Autodesk Inventor part; units mm, degrees
ref_plane "YZ Plane" through (0, 0, 0) normal (1, 0, 0) x (0, 1, 0)
ref_plane "XZ Plane" through (0, 0, 0) normal (0, 1, 0) x (-1, 0, 0)
ref_plane "XY Plane" through (0, 0, 0) normal (0, 0, 1) x (1, 0, 0)
sketch "Sketch1" plane through (0, 0, 0) normal (1, 0, 0) x (0, 1, 0)
  circle A0 centre (0, 0) radius 3
  circle A1 centre (0, 77) radius 3
  circle A2 centre (36, 77) radius 3
  line L0 (-5, 78) -> (-5, -1)
  line L1 (-1, 82) -> (37, 82)
  line L2 (41, 78) -> (41, 76)
  line L3 (37, 72) -> (9, 72)
  line L4 (5, 68) -> (5, -1)
  line L5 (36, 77) -> (41, 77)
  line L6 (0, 0) -> (0, -5)
  line L7 (0, -5) -> (1, -5)
  line L8 (-1, -5) -> (0, -5)
  arc A3 (-1, 82) -> (-5, 78) centre (-1, 78) ccw
  arc A4 (-5, -1) -> (-1, -5) centre (-1, -1) ccw
  arc A5 (1, -5) -> (5, -1) centre (1, -1) ccw
  arc A6 (9, 72) -> (5, 68) centre (9, 68) ccw
  arc A7 (37, 72) -> (41, 76) centre (37, 76) ccw
  arc A8 (41, 78) -> (37, 82) centre (37, 78) ccw
  dimension "d0" = 6
  dimension "d1" = 77
  dimension "d3" = 10
  dimension "d4" = 5
  dimension "d5" = 4
  dimension "d6" = 10
  dimension "d9" = 46
extrude "Extrusion1" add sketch "Sketch1" along normal blind 19
sketch "Sketch3" plane through (0, 5, -1) normal (0, 1, 0) x (1, 0, 0)
  line L0 (19, 0) -> (19, -69)
  line L1 (19, -27) -> (0, -27)
  line L2 (0, -27) -> (0, -54)
  line L3 (0, -54) -> (19, -54)
  line L4 (19, -54) -> (19, -27)
  line L5 (0, 4) -> (19, 4)
  line L6 (0, -83) -> (19, -83)
  line L7 (0, 0) -> (0, -69)
  point P0 (0, -1)
  point P1 (19, -54)
  dimension "d15" = 31
  dimension "d16" = 29
extrude "Extrusion3" add sketch "Sketch3" along normal blind 8
fillet "Fillet1" radius 4 2 edges at (9.5, 5, 53) (9.5, 5, 26)
sketch "Sketch4" plane through (0, 5, -1) normal (0, 1, 0) x (1, 0, 0)
  line L0 (12.5, -15.2321) -> (9.5, -16.9641)
  line L1 (9.5, -16.9641) -> (6.5, -15.2321)
  line L2 (6.5, -15.2321) -> (6.5, -11.7679)
  line L3 (6.5, -11.7679) -> (9.5, -10.0359)
  line L4 (9.5, -10.0359) -> (12.5, -11.7679)
  line L5 (12.5, -11.7679) -> (12.5, -15.2321)
  line L6 (12.5, -65.2321) -> (9.5, -66.9641)
  line L7 (9.5, -66.9641) -> (6.5, -65.2321)
  line L8 (6.5, -65.2321) -> (6.5, -61.7679)
  line L9 (6.5, -61.7679) -> (9.5, -60.0359)
  line L10 (9.5, -60.0359) -> (12.5, -61.7679)
  line L11 (12.5, -61.7679) -> (12.5, -65.2321)
  line L12 (19, -58) -> (19, -69)
  line L13 (19, 0) -> (19, -23)
  line L14 (19, -23) -> (0, -23)
  line L15 (19, -27) -> (0, -27)
  line L16 (0, -54) -> (19, -54)
  circle A0 centre (9.5, -13.5) radius 1.5
  circle A1 centre (9.5, -63.5) radius 1.5
  point P0 (0, -1)
  point P1 (9.5, -23)
  dimension "d20" = 6
  dimension "d23" = 9.5
  dimension "d26" = 3
  dimension "d29" = 50
extrude "Extrusion4" cut sketch "Sketch4" against normal blind 3 contours L0 L1 L2 L3 L4 L5 | L6 L7 L8 L9 L10 L11 | A0 | A1
extrude "Extrusion5" cut sketch "Sketch4" against normal through all contours A0 | A1
sketch "Sketch5" plane through (0, 13, -1) normal (0, 1, 0) x (1, 0, 0)
  circle A0 centre (5.5, -31.8771) radius 1.25
  circle A1 centre (5.5, -48.8771) radius 1.25
  circle A2 centre (13.5, -31.8771) radius 1.25
  circle A3 centre (13.5, -48.8771) radius 1.25
  line L0 (19, -54) -> (19, -27)
  line L1 (0, -27) -> (0, -54)
  point P0 (0, -1)
  dimension "d30" = 2.5
  dimension "d31" = 17
  dimension "d32" = 5.5
  dimension "d33" = 5.5
extrude "Extrusion6" cut sketch "Sketch5" against normal through all
equation "\"d33\" = d32"
properties part number "wheel_mount"
Verification items for the finished model (mm, model axes). A direction names the side the tool comes from. Give positions to 0.01 mm unless a question says otherwise; leave off trailing zeros. Order: outer loops, then holes, each group sorted by start corner. A loop starts at its lowest first (then second) coordinate and runs counter-clockwise, first axis right, second up. Notation, with made-up numbers: (38.5, -36.5) - (58.5, -36.5) arc R7 cw to (58.5, -25.5) - close; hole circle Ø4 at (63, 87). An arc over 180 degrees is marked (long way). Answer as CSV lines item,"result". Start each with the question number.
Item 1: Access from +Z, -Z, +X, -X, +Y, -Y to the whole of each face (thin tool, end or side, straight path). Record for faces 1 (the face through (0, 6, 45)), 2 (the face through (10, 11, 26)), 3 (the face through (9, 41, 77)), 4 (the face through (8, 3.5, 59.9)), 5 (the face through (9.633, 6.141, 54.203)).
Item 2: Section check D-D, the plane x = 16. Record the boundary of the cut face in (y, z).
Item 3: Mould release check, pull along Z, two halves, no side actions. Record for faces 6 (the face through (9.37, -0.65, 79.93)), 7 (the face through (8, -1.45, 12.43)), 8 (the face through (9, 5, 8)), 9 (the face through (9.367, 6.141, 24.797)): released by +Z, released by -Z, zero draft, split by the parting line, or undercut.
Item 4: Material ranges on L1, parallel to Z at x = 15.25, y = 0; L2, parallel to Z at x = 9.5, y = -2.25; L3, parallel to Z at x = 5.5, y = 3.75, recorded low to high.
Item 5: Section check A-A, the plane x = 5.5. State how many separate pieces and enclosed holes the cut face has, plus the area to 3 significant figures.
Item 6: Gauge pin test, flat ends, axial feed: pin 1 (3.5 mm diameter, centred on x = 11.5, z = 60.5, fed in from +Y); pin 2 (2 mm diameter, centred on x = 13.5, z = 30.88, fed in from +Y); pin 3 (1.2 mm diameter, centred on x = 9, y = 11, fed in from -Z); pin 4 (3 mm diameter, centred on x = 13.5, z = 47.88, fed in from +Y). Record the tip position at first contact, or that the pin passes through.
Item 7: Section check B-B, the plane z = 62.5. Record the boundary of the cut face in (x, y).
Item 8: Section check C-C, the plane y = 36. Record the boundary of the cut face in (x, z).
Filled in:
1,face 1,"+Z, -Z, -X, +Y, -Y"
1,face 2,"-Z, +X, -X, +Y"
1,face 3,"+Z, -Z, +X, -X, +Y"
1,face 4,"+Y"
1,face 5,"+X, -X, +Y"
2,outline,"(-5, -1) arc R4 ccw to (-1, -5) - (1, -5) arc R4 ccw to (5, -1) - (5, 22) arc R4 cw to (9, 26) - (13, 26) - (13, 53) - (9, 53) arc R4 cw to (5, 57) - (5, 68) arc R4 cw to (9, 72) - (37, 72) arc R4 ccw to (41, 76) - (41, 78) arc R4 ccw to (37, 82) - (-1, 82) arc R4 ccw to (-5, 78) - close; hole circle Ø6 at (0, 0); hole circle Ø6 at (0, 77); hole circle Ø6 at (36, 77)"
3,face 6,"undercut"
3,face 7,"undercut"
3,face 8,"zero draft"
3,face 9,"released by -Z"
4,L1,"-5 to -3, 3 to 74, 80 to 82"
4,L2,"-4.8 to -1.98, 1.98 to 11, 14 to 61, 64 to 75.02, 78.98 to 81.8"
4,L3,"-3.9 to 29.63, 32.13 to 46.63, 49.13 to 82"
5,separate pieces,"3"
5,enclosed holes,"3"
5,area,"1,260 mm^2"
6,pin 1,"y = 5"
6,pin 2,"through"
6,pin 3,"z = 26"
6,pin 4,"y = 13"
7,outline,"(0, -5) - (8, -5) - (8, 2) - (6.5, 2) - (6.5, 5) - (0, 5) - close; (11, -5) - (19, -5) - (19, 5) - (12.5, 5) - (12.5, 2) - (11, 2) - close"
8,outline,"(0, 72) - (19, 72) - (19, 74) - (0, 74) - close; (0, 80) - (19, 80) - (19, 82) - (0, 82) - close"
